Source: CAD feature listing. Evaluate the final solid. Frame: model axes, mm. A direction names the side the tool comes from. Coordinates: 2 decimals unless noted, no trailing zeros. Order: outer loops, then holes, each group sorted by start corner. A loop starts at its lowest first (then second) coordinate and runs counter-clockwise, first axis right, second up. Notation, with made-up numbers: (30, 11) -> (81, 11) arc R10 cw to (81, 17) -> close; hole circle Ø6 at (31.25, 51.5). An arc over 180 degrees is marked (long way). Write item = value, one per line. Start each with the question number.
Item 1: Section query C-C (x = 7.75). Output: boundary loops of the cut face in (y, z).
Item 2: Set-up query: faces 1 (the cylindrical face through (5, 0, 2)), 2 (the cylindrical face through (0.478, -0.387, 1.743)), 3 (the flat face through (-2.6, 2, 0)), 4 (the flat face through (-1.5, 0, 0)), 5 (the flat face through (10, 0, 0)). Return all of +Z, -Z, +X, -X, +Y, -Y with unobstructed straight access to the full face (end or side cutting, diameter ignored); none if empty.
Item 3: Contact query for flat-ended pins moving along their axis: pin 1 (4 mm diameter, centred on x = 4.5, z = -2, fed in from -Y); pin 2 (3 mm diameter, centred on x = 0.5, y = -2.5, fed in from -Z); pin 3 (1.2 mm diameter, centred on x = -2, z = -1.5, fed in from +Y); pin 4 (2 mm diameter, centred on y = 1, z = -1.5, fed in from +X). Output: stop coordinate, or through.
Item 4: Mould query, pull axis Y, two halves, no side actions, for faces 6 (the conical face through (-1.46, 1.56, -2.99)), 7 (the flat face through (-2, -0.6, 0)), 8 (the flat face through (-2.6, -2, 0)). Classes: released by +Y, released by -Y, zero draft, split by the parting line, or undercut.
Item 5: Section query D-D (x = -1). Output: boundary loops of the cut face in (y, z) (1 decimal).
Item 6: Section query B-B (y = 0). Output: boundary loops of the cut face in (x, z), then the cut area to 3 significant figures.
Item 7: Ray query, line 1 along X through (y, z) = (2.75, 0.75); line 2 along X through (y, z) = (-0.5, 0.75); line 3 along Z through (x, y) = (6.75, 0). Return the intervals inside material, ascending. Write a range as [from, to].
Item 8: Section query A-A (z = 0). Output: boundary loops of the cut face in (x, y).
Autodesk Inventor part; units mm, degrees
ref_plane "Work Plane1" through (30.1625, 0, 0) normal (0, 0, -1) x (1, 0, 0)
ref_plane "YZ Plane" through (0, 0, 0) normal (1, 0, 0) x (0, 1, 0)
ref_plane "XZ Plane" through (0, 0, 0) normal (0, 1, 0) x (-1, 0, 0)
sketch "Sketch1" plane through (0, 0, 0) normal (0, 0, 1) x (1, 0, 0)
  line L0 (-2.6, 0) -> (10, 0)
  line L1 (10, 0) -> (10, 2)
  line L2 (10, 2) -> (1.4, 2)
  line L3 (1.4, 2) -> (0.9705, 1.7853)
  line L4 (0.9705, 1.7853) -> (0, 1.7853)
  line L5 (0, 1.7853) -> (0, 3.5)
  line L6 (-5.12, 0) -> (12.52, 0)
  line L7 (0, -0.7) -> (0, 4.2)
  line L8 (-2.6, 0) -> (-2.6, 3.2725)
  line L9 (0, 3.5) -> (-2.6, 3.2725)
  line L10 (1.4, 2) -> (0, 2) construction
  dimension "d0" = 10
  dimension "d1" = 8.6
  dimension "d2" = 0.4295
  dimension "d3" = 2.6
  dimension "d4" = 4
  dimension "d5" = 3.5705
  dimension "d9" = 7
  dimension "d10" = 5
revolve "Body" add sketch "Sketch1" angle 360 about axis through (-2.6, 0, 0) along (1, 0, 0)
sketch "Sketch2" plane through (-2.6, 0, 0) normal (-1, 0, 0) x (0, 0, 1)
  circle A0 centre (0, 0) radius 3.5
  line L0 (0, 0) -> (0, 3.2725)
  line L1 (-3.5, 0.6) -> (3.5, 0.6)
  line L2 (3.5, 0.6) -> (3.5, -0.6)
  line L3 (3.5, -0.6) -> (-3.5, -0.6)
  line L4 (-3.5, -0.6) -> (-3.5, 0.6)
  line L5 (-3.5, 0) -> (3.5, 0) construction
  line L6 (0, 0.6) -> (0, -0.6) construction
  dimension "d11" = 1.2
  dimension "d12" = 7
fillet "Fillet1" radius 0.2 1 edges at (-2.6, -3.2725, 0)
extrude "Slot" cut sketch "Sketch2" against normal blind 1.1 contours A0 L3 L1 | L2 L3 A0 | A0 L1 L2 | A0 L4 L1 | L3 L4 A0
thread "Thread"
chamfer "Chamfer1" distance 0.4294 distance2 0.4295 1 edges at (10, -2, 0) measured on face at (10, -0.6816, 0.4421)
ref_plane "Work Plane1" through (30.1625, 0, 0) normal (0, 0, -1) x (1, 0, 0)
equation "\"d11\" = SBR"
equation "\"d12\" = KOD"
equation "\"d19\" = STI"
equation "\"d14\" = RR"
equation "\"d15\" = GEL"
equation "\"d17\" = -0.5 * SPD + 0.5 * GD"
equation "\"d0\" = NLG"
equation "\"d1\" = GEL"
equation "\"d3\" = KOH"
equation "\"d4\" = GD"
equation "\"d5\" = BDM"
equation "\"d9\" = KOD"
equation "\"d10\" = KEWI"
equation "\"GD\" = NND"
equation "\"NLG\" = 10"
equation "\"GEL\" = 8.6"
equation "\"KOD\" = 7"
equation "\"KOH\" = 2.6"
equation "\"GAL\" = 0.61345 * PTC"
equation "\"SPD\" = NND - 1.2269 * PTC"
equation "\"BDM\" = 3.5705"
equation "\"GUL\" = 0.61345 * PTC"
equation "\"RR\" = 0.2"
equation "\"SBR\" = 1.2"
equation "\"STI\" = 1.1"
equation "\"KEWI\" = 5deg"
equation "\"PTC\" = 0.7"
equation "\"THREADDIA\" = 4"
equation "\"TOA\" = 30deg"
equation "\"NND\" = 4"
equation "\"GD1\" = THREADDIA - 1.2269 * PTC"
properties part number "ISO 1207 - M4 x 10" material "Stainless Steel, 440C"
Computed:
q1.outline = circle Ø4 at (0, 0)
q2.face_1 = +X
q2.face_2 = none
q2.face_3 = +Z, -Z, -X, +Y, -Y
q2.face_4 = +Z, -Z, -X
q2.face_5 = +Z, -Z, +X, +Y, -Y
q3.pin_1 = -2
q3.pin_2 = -3.33
q3.pin_3 = 3.21
q3.pin_4 = 10
q4.face_6 = split by the parting line
q4.face_7 = undercut
q4.face_8 = zero draft
q5.outline = circle Ø6.8 at (0, 0)
q6.outline = (-1.5, -3.37) -> (0, -3.5) -> (0, -1.79) -> (0.97, -1.79) -> (1.4, -2) -> (9.57, -2) -> (10, -1.57) -> (10, 1.57) -> (9.57, 2) -> (1.4, 2) -> (0.97, 1.79) -> (0, 1.79) -> (0, 3.5) -> (-1.5, 3.37) -> close
q6.area = 49.6 mm^2
q7.line_1 = [-2.6, 0]
q7.line_2 = [-1.5, 10]
q7.line_3 = [-2, 2]
q8.outline = (-2.6, -3.09) arc R0.2 ccw to (-2.42, -3.29) -> (0, -3.5) -> (0, -1.79) -> (0.97, -1.79) -> (1.4, -2) -> (9.57, -2) -> (10, -1.57) -> (10, 1.57) -> (9.57, 2) -> (1.4, 2) -> (0.97, 1.79) -> (0, 1.79) -> (0, 3.5) -> (-2.42, 3.29) arc R0.2 ccw to (-2.6, 3.09) -> (-2.6, 0.6) -> (-1.5, 0.6) -> (-1.5, -0.6) -> (-2.6, -0.6) -> close
